Autodesk Inventor part; units mm, degrees
ref_plane "YZ Plane" through (0, 0, 0) normal (1, 0, 0) x (0, 1, 0)
ref_plane "XZ Plane" through (0, 0, 0) normal (0, 1, 0) x (-1, 0, 0)
ref_plane "XY Plane" through (0, 0, 0) normal (0, 0, 1) x (1, 0, 0)
sketch "Sketch1" plane through (0, 0, 0) normal (0, 0, 1) x (1, 0, 0)
  line L0 (-28, 5) -> (28, 5)
  line L1 (28, 5) -> (28, -5)
  line L2 (28, -5) -> (-28, -5)
  line L3 (-28, -5) -> (-28, 5)
  line L4 (-10, 30) -> (10, 30)
  line L5 (10, 30) -> (10, 5)
  line L6 (10, 5) -> (-10, 5)
  line L7 (-10, 5) -> (-10, 30)
  circle A0 centre (0, 22) radius 5.15
  line L8 (-1.5, 30) -> (1.5, 30)
  line L9 (1.5, 30) -> (1.5, 8)
  line L10 (1.5, 8) -> (-1.5, 8)
  line L11 (-1.5, 8) -> (-1.5, 30)
  point P0 (0, 0)
  point P1 (-28, 0)
  point P2 (0, 5)
  point P3 (0, 30)
  point P4 (0, 30)
  point P5 (-1.5, 17.0733)
  point P6 (-1.5, 26.9267)
  point P7 (-1.5, 30)
  point P8 (-10, 5)
  point P9 (10, 5)
  point P10 (1.5, 30)
  point P11 (1.5, 26.9267)
  point P12 (1.5, 17.0733)
  dimension "d0" = 10
  dimension "d1" = 20
  dimension "d2" = 10.3
  dimension "d3" = 17
  dimension "d4" = 8
  dimension "d5" = 3
  dimension "d6" = 14
  dimension "d7" = 18
extrude "Extrusion1" add sketch "Sketch1" along normal mid plane 20 contours L0 L1 L2 L3 | L7 L4 L11 A0 L10 L9 L5 L0
sketch "Sketch2" plane through (10, 5, 10) normal (0, 1, 0) x (1, 0, 0)
  line L0 (0, 20) -> (18, 20)
  line L1 (-38, 20) -> (-20, 20)
  line L2 (-38, 20) -> (-38, 0)
  line L3 (18, 20) -> (18, 0)
  point P0 (-10, 10)
  point P1 (-31, 10)
  point P2 (11, 10)
  point P3 (9, 20)
  point P4 (-38, 10)
  point P5 (18, 10)
  dimension "d29" = 7
  dimension "d30" = 7
hole "Hole1" at (-21, 5, 0) at (21, 5, 0) direction (0, -1, 0) diameter 6 end through all
sketch "Sketch4" plane through (0, 0, 10) normal (0, 0, 1) x (1, 0, 0)
  line L0 (-10, 5) -> (-28, 5)
  line L1 (-28, 5) -> (-28, -5)
  line L2 (-28, -5) -> (28, -5)
  line L3 (28, -5) -> (28, 5)
  line L4 (28, 5) -> (10, 5)
  line L5 (10, 5) -> (10, 30)
  line L6 (10, 30) -> (1.5, 30)
  line L7 (1.5, 30) -> (1.5, 26.9267)
  arc A0 (1.5, 17.0733) -> (1.5, 26.9267) centre (0, 22) ccw
  line L8 (1.5, 17.0733) -> (1.5, 8)
  line L9 (1.5, 8) -> (-1.5, 8)
  line L10 (-1.5, 8) -> (-1.5, 17.0733)
  arc A1 (-1.5, 26.9267) -> (-1.5, 17.0733) centre (0, 22) ccw
  line L11 (-1.5, 26.9267) -> (-1.5, 30)
  line L12 (-1.5, 30) -> (-10, 30)
  line L13 (-10, 30) -> (-10, 5)
  line L14 (-10, 5) -> (-28, 5)
  line L15 (28, 5) -> (10, 5)
  line L16 (-10, 5) -> (10, 5)
  point P0 (0, 0)
extrude "Extrusion3" add sketch "Sketch4" along normal blind 30 contours L16 L4 L3 L2 L1 L0
sketch "Sketch3" plane through (10, 5, 10) normal (1, 0, 0) x (0, 0, -1)
  line L0 (20, 25) -> (0, 25)
  circle A0 centre (10, 7.0733) radius 2.75
  line L1 (20, 25) -> (0, 25)
  line L2 (0, 25) -> (8, 25)
  line L3 (8, 25) -> (8, 0)
  line L4 (8, 0) -> (0, 0)
  line L5 (0, 0) -> (0, 25)
  line L6 (20, 0) -> (0, 0)
  line L7 (12, 25) -> (20, 25)
  line L8 (20, 25) -> (20, 0)
  line L9 (20, 0) -> (12, 0)
  line L10 (12, 0) -> (12, 25)
  line L11 (20, 25) -> (20, 0)
  line L12 (20, 12.0733) -> (0, 12.0733)
  point P0 (10, -5)
  point P1 (10, 25)
  point P2 (12, 0)
  dimension "d18" = 5.5
  dimension "d19" = 8
  dimension "d21" = 8
  dimension "d31" = 5
extrude "Extrusion2" cut sketch "Sketch3" against normal through all contours L10 A0 L3 | A0 L10 | L3 A0
sketch "Sketch5" plane through (-10, 5, 10) normal (0, 1, 0) x (-1, 0, 0)
  circle A0 centre (6.1591, 21.8725) radius 1.7875
  circle A1 centre (-13.0159, 21.8725) radius 1.7875
  point P0 (-10, -10)
extrude "Extrusion4" cut sketch "Sketch5" against normal blind 10
equation "\"d21\" = d19"
properties part number "0008-10-052 Suport Axa Y +Senzor"
Design review of the part built by this model. Coordinates are the model's own, in mm. A direction names the side the tool comes from. Coordinates: 2 decimals unless noted, no trailing zeros. Loops run counter-clockwise (first coordinate to the right, second up) from the corner with the lowest first, then second, coordinate; pieces in that order, holes last.
Q1. To check wall thickness, follow line 1 (Y direction, x = 4, z = 0); line 2 (Z direction, x = 21, y = 0); line 3 (X direction, y = 0.5, z = 0). State the ranges of each line that lie inside material, in increasing order.
Reported:
line 1: y = -5 to 9.32, 14.82 to 18.76, 25.24 to 30
line 2: z = -10 to -3, 3 to 40
line 3: x = -28 to -24, -18 to 18, 24 to 28
Q2. We need section D-D on x = -7. State the section outline as (y, z) points.
Reported:
outline: (-5, -10) - (30, -10) - (30, 10) - (5, 10) - (5, 40) - (-5, 40) - close; hole circle Ø5.5 at (12.07, 0)
Q3. We need section B-B on x = -21. State the section outline as (y, z) points.
Reported:
outline: (-5, -10) - (5, -10) - (5, -3) - (-5, -3) - close; (-5, 3) - (5, 3) - (5, 40) - (-5, 40) - close
Q4. For pin 1 (5 mm diameter, centred on x = 21, z = 0, fed in from +Y) (1 decimal); pin 2 (10 mm diameter, centred on x = -2.5, y = 23, fed in from +Z); pin 3 (8 mm diameter, centred on x = 14.5, z = 26, fed in from +Y); pin 4 (0.9 mm diameter, centred on y = 27.5, z = 0, fed in from +X), all flat-tipped, find the tip position at first contact; note any pin that passes through.
Reported:
pin 1: passes through
pin 2: stops at z = 10
pin 3: stops at y = 5
pin 4: stops at x = 10
Q5. We need section A-A on z = 0. State how many separate pieces and enclosed holes the cut face has, and give its area (3 significant figures).
Reported:
separate pieces: 5
enclosed holes: 0
area: 728 mm2
Q6. The part is to be moulded in two halves that separate along Z. For faces 5 (the face through (5.81, 9.39, 0.6)), 6 (the face through (0, 5, 15)), 7 (the face through (0, 5, -10)), 8 (the face through (0, 0, 40)), say which applies: +Z half, -Z half, draft (parallel to the pull), parting line (faces both ways), or undercut.
Reported:
face 5: undercut
face 6: draft
face 7: -Z half
face 8: +Z half
Q7. We need section C-C on y = 20.5. State the section outline as (x, z) points.
Reported:
outline: (-10, -10) - (-4.93, -10) - (-4.93, 10) - (-10, 10) - close; (4.93, -10) - (10, -10) - (10, 10) - (4.93, 10) - close
Q8. Tool access review of faces 1 (the face through (-10, 17, 0)), 2 (the face through (1.5, 28, 0)), 3 (the face through (-5.15, 21.91, -0.14)), 4 (the face through (-2, 15, 10)): name each direction out of +Z, -Z, +X, -X, +Y, -Y from which nothing blocks a thin tool from reaching the whole face with its end or side.
Reported:
face 1: +Z, -Z, -X, +Y
face 2: +Z, -Z, +Y
face 3: +Z, -Z
face 4: +Z, +X, -X, +Y
